Autodesk Inventor part; units mm, degrees
ref_plane "YZ Plane" through (0, 0, 0) normal (1, 0, 0) x (0, 1, 0)
ref_plane "XZ Plane" through (0, 0, 0) normal (0, 1, 0) x (-1, 0, 0)
ref_plane "XY Plane" through (0, 0, 0) normal (0, 0, 1) x (1, 0, 0)
sketch "Skizze1" plane through (0, 0, 0) normal (0, 0, 1) x (1, 0, 0)
  circle A0 centre (0, 0) radius 15
  circle A1 centre (0, 0) radius 17.5
  dimension "d0" = 35
  dimension "d1" = 2.5
extrude "Extrusion1" add sketch "Skizze1" along normal blind 250
sketch "Skizze2" plane through (0, 0, 250) normal (0, 0, 1) x (1, 0, 0)
  circle A0 centre (0, 0) radius 17.5
  circle A1 centre (0, 0) radius 17
  dimension "d4" = 34
extrude "Extrusion2" cut sketch "Skizze2" against normal through all
sketch "Skizze3" plane through (0, 0, 0) normal (0, 0, -1) x (-1, 0, 0)
  circle A0 centre (0, 0) radius 17
  circle A1 centre (0, 0) radius 15
  circle A2 centre (0, 0) radius 17.5
  dimension "d7" = 35
extrude "Extrusion3" add sketch "Skizze3" against normal blind 9 contours A2
sketch "Skizze4" plane through (0, 0, 250) normal (0, 0, 1) x (1, 0, 0)
  circle A0 centre (0, 0) radius 17
  circle A1 centre (0, 0) radius 15
  circle A2 centre (0, 0) radius 16.5
  dimension "d10" = 33
extrude "Extrusion4" cut sketch "Skizze4" against normal blind 50 contours A0
sketch "Skizze5" plane through (0, 0, 0) normal (0, 1, 0) x (-1, 0, 0)
  line L0 (-17.5, 9) -> (17.5, 9)
  line L1 (17.5, 0) -> (-17.5, 0)
  line L2 (17, 9) -> (-17, 9)
  line L3 (17.5, 0) -> (17.5, 9)
  line L4 (15, 0) -> (15, 250)
  line L5 (17, 200) -> (17, 9)
  line L6 (17.5, 9) -> (16.75, 9)
  line L7 (16.75, 9) -> (16.75, 7)
  line L8 (16.75, 7) -> (17.5, 7)
  line L9 (17.5, 7) -> (17.5, 9)
  line L10 (24.5, 0) -> (-24.5, 0)
  line L11 (0, -50) -> (0, 300)
  point P0 (0, 0)
  point P1 (-9.75, 200)
  point P2 (9.75, 200)
  dimension "d13" = 2
  dimension "d14" = 33.5
revolve "Umdrehung1" cut sketch "Skizze5" angle 360 about axis through (0, 0, -10) along (0, 0, 1) contours L0 L3 L8 L7
chamfer "Fase1" distance 0.75 angle 45 1 edges at (17.5, 0, 7)
thread "Gewinde5"
sketch "Skizze6" plane through (0, 0, 200) normal (0, 0, 1) x (1, 0, 0)
  circle A0 centre (0, 0) radius 16.5
  circle A1 centre (0, 0) radius 17
extrude "Extrusion5" add sketch "Skizze6" along normal blind 50
properties part number "13_0204_027"
Can you work these out from the model? Positions are in its coordinate system, mm. A direction names the side the tool comes from. Round coordinates to 2 decimals unless told otherwise and drop trailing zeros. Write each loop counter-clockwise with the first axis right and the second up, starting at its lowest first coordinate (ties: lowest second). Pieces come first, ordered by that corner, then holes. Notation, with made-up numbers: (58, 87.25) - (87, 87.25) arc R27 cw to (87, 114.25) - close; hole circle Ø4 at (76, -6.5). An arc over 180 degrees is marked (long way). Write each question's results on one line, items separated by ' | '. Start each with the question number.
1) We'd pull the mould along Z, two halves only. Please class faces 3 (the cylindrical face through (3.63, -16.35, 7.99)), 4 (the cylindrical face through (13.887, -10.648, 3.081)), 5 (the flat face through (-13, 8, 0)): released by +Z, released by -Z, zero draft, split by the parting line, or undercut.
2) Suppose I cut it at C-C (z = 234). List the corners of the cut face in (x, y) for me.
3) Which directions (+Z, -Z, +X, -X, +Y, -Y) give clear straight access to the entire face, cutting with the end or side of a thin tool? Please do faces 1 (the cylindrical face through (9.139, -14.334, 127.813)), 2 (the flat face through (6, -14, 250)).
4) Please list where these lines run through material, in increasing order: line 1 (Y direction, x = 0, z = 190.5); line 2 (X direction, y = -0.5, z = 167); line 3 (X direction, y = -7, z = 67.5).
5) For pin 1 Ø2 at (x, z) = (11.5, 32.5) entering from -Y; pin 2 Ø8 at (x, z) = (4.5, 30.5) entering from +Y; pin 3 Ø2 at (y, z) = (-2.5, 92) entering from -X, each with a flat end and sliding along its axis, tell me the tip position at first contact or that it passes through.
Here are the results:
1) face 3: undercut | face 4: zero draft | face 5: released by -Z
2) outline: circle Ø34 at (0, 0); hole circle Ø30 at (0, 0)
3) face 1: +Z | face 2: +Z, +X, -X, +Y, -Y
4) line 1: y = -17 to -15, 15 to 17 | line 2: x = -16.99 to -14.99, 14.99 to 16.99 | line 3: x = -15.49 to -13.27, 13.27 to 15.49
5) pin 1: stops at y = -13.37 | pin 2: stops at y = 16.99 | pin 3: stops at x = -16.93
